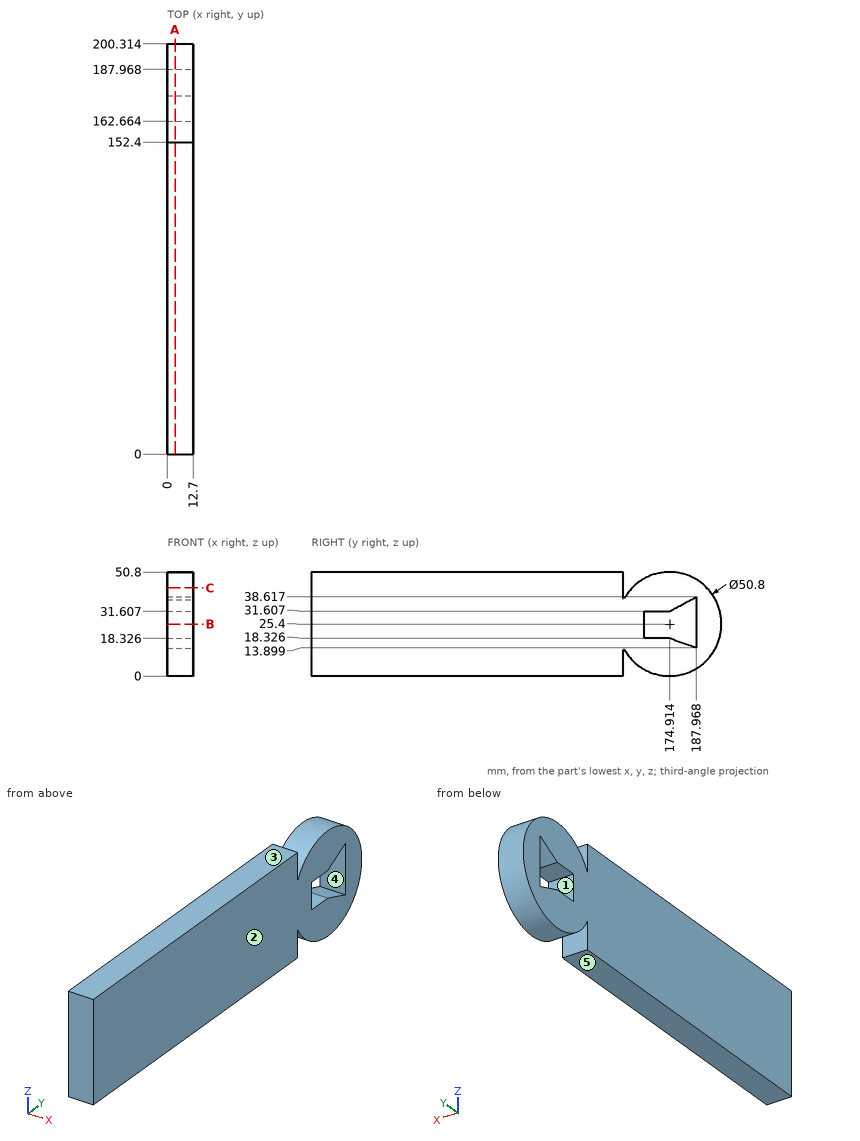
Verification items for this drawing (mm, ordinates from the low corner). A direction names the side the tool comes from. Give positions to 0.01 mm unless a question says otherwise; leave off trailing zeros. Write each loop counter-clockwise with the first axis right and the second up, starting at its lowest first coordinate (ties: lowest second). Pieces come first, ordered by that corner, then holes.
1) Release check for a two-part mould opening along Z. For the marked faces 1, 2 and 3 record: pulls with the +Z half, pulls with the -Z half, needs draft (parallel to the pull), parting line crosses it, or undercut.
2) Section check A-A, the plane x = 3.75. Record the boundary of the cut face in (y, z).
3) Material ranges on L1, parallel to Z at x = 1.75, y = 174.5; L2, parallel to Y at x = 9.5, z = 48 (1 decimal); L3, parallel to Z at x = 8.75, y = 182, recorded low to high.
4) Gauge pin test, flat ends, axial feed: pin 1 (3.5 mm diameter, centred on x = 8, y = 168, fed in from +Z); pin 2 (3 mm diameter, centred on x = 6.5, z = 31.5, fed in from +Y). Record the tip position at first contact, or that the pin passes through.
5) Section check C-C, the plane z = 43. Record the boundary of the cut face in (x, y), and give its area (3 significant figures).
6) Section check B-B, the plane z = 25.4. Record the boundary of the cut face in (x, y).
7) Access from +Z, -Z, +X, -X, +Y, -Y to the whole of each face (thin tool, end or side, straight path). Record for the marked faces 4 and 5.
Computed:
1. face 1: undercut
1. face 2: needs draft
1. face 3: pulls with the +Z half
2. outline: (0, 0) - (152.4, 0) - (152.4, 13.64) arc R25.4 ccw (long way) to (152.4, 37.16) - (152.4, 50.8) - (0, 50.8) - close; hole (162.66, 18.33) - (174.91, 18.33) - (187.97, 13.9) - (187.97, 38.62) - (174.91, 31.61) - (162.66, 31.61) - close
3. L1: z = 0 to 18.33, 31.61 to 50.8
3. L2: y = 0 to 152.4, 163.3 to 186.5
3. L3: z = 1.01 to 15.92, 35.41 to 49.79
4. pin 1: stops at z = 50.27
4. pin 2: stops at y = 199.89
5. outline: (0, 0) - (12.7, 0) - (12.7, 152.4) - (0, 152.4) - close; (0, 156.6) - (12.7, 156.6) - (12.7, 193.23) - (0, 193.23) - close
5. area: 2,400 mm2
6. outline: (0, 0) - (12.7, 0) - (12.7, 162.66) - (0, 162.66) - close; (0, 187.97) - (12.7, 187.97) - (12.7, 200.31) - (0, 200.31) - close
7. face 4: +X, -X
7. face 5: -Z, +X, -X, +Y, -Y
